```python
from build123d import *

# Parameters (mm, degrees)
F0_W     = 76.2
F0_H     = 50.8
F1_DEPTH = 12.7
F3_DEPTH = 50.801
F5_DEPTH = 76.201
F6_R     = 1.27
F7_DEPTH = 12.701


# Not quite as in the source:
# - a feature names something its author has since deleted; it is built from what else it names


with BuildPart() as f1:
    # F0 (on Top) → F1 (new body)
    with BuildSketch(Plane.XY):
        Rectangle(F0_W, F0_H)
    extrude(amount=F1_DEPTH)

    # F2 (on face) → F3 (cut, through all)
    with BuildSketch(Plane.XZ.offset(25.4)):
        with BuildLine():
            Line((6.4135, 12.7), (-6.4135, 12.7))
            Line((-6.4135, 12.7), (-6.4135, 11.2776))
            ThreePointArc((-6.4135, 11.2776), (-5.7912, 10.6553), (-6.4135, 10.033))
            Line((-6.4135, 10.033), (-6.4135, 8.7376))
            ThreePointArc((-6.4135, 8.7376), (-5.7912, 8.1153), (-6.4135, 7.493))
            Line((-6.4135, 7.493), (-6.4135, 6.223))
            Line((-6.4135, 6.223), (6.4135, 6.223))
            Line((6.4135, 6.223), (6.4135, 7.493))
            ThreePointArc((6.4135, 7.493), (5.7912, 8.1153), (6.4135, 8.7376))
            Line((6.4135, 8.7376), (6.4135, 10.033))
            ThreePointArc((6.4135, 10.033), (5.7912, 10.6553), (6.4135, 11.2776))
            Line((6.4135, 11.2776), (6.4135, 12.7))
        make_face()
    extrude(amount=-F3_DEPTH, mode=Mode.SUBTRACT)

    # F4 (on face) → F5 (cut, through all)
    with BuildSketch(Plane.YZ.offset(38.1)):
        with BuildLine():
            Line((6.4135, 12.7), (-6.4135, 12.7))
            Line((-6.4135, 12.7), (-6.4135, 11.2776))
            ThreePointArc((-6.4135, 11.2776), (-5.7912, 10.6553), (-6.4135, 10.033))
            Line((-6.4135, 10.033), (-6.4135, 8.7376))
            ThreePointArc((-6.4135, 8.7376), (-5.7912, 8.1153), (-6.4135, 7.493))
            Line((-6.4135, 7.493), (-6.4135, 6.223))
            Line((-6.4135, 6.223), (6.4135, 6.223))
            Line((6.4135, 6.223), (6.4135, 7.493))
            ThreePointArc((6.4135, 7.493), (5.7912, 8.1153), (6.4135, 8.7376))
            Line((6.4135, 8.7376), (6.4135, 10.033))
            ThreePointArc((6.4135, 10.033), (5.7912, 10.6553), (6.4135, 11.2776))
            Line((6.4135, 11.2776), (6.4135, 12.7))
        make_face()
    extrude(amount=-F5_DEPTH, mode=Mode.SUBTRACT)

    # F6 (on Top) → F7 (cut, through all)
    with BuildSketch(Plane.XY):
        Circle(F6_R)
    extrude(amount=F7_DEPTH, mode=Mode.SUBTRACT)


solid = f1.part
```
Design review of the part built by this model. Coordinates are the model's own, in mm. A direction names the side the tool comes from. Round coordinates to 2 decimals unless told otherwise and drop trailing zeros. Write each loop counter-clockwise with the first axis right and the second up, starting at its lowest first coordinate (ties: lowest second). Pieces come first, ordered by that corner, then holes.
Item 1: We need section D-D on y = -19. Write out the cut boundary in (x, z), and give its area (3 significant figures).
Item 2: We need section B-B on y = 0. Write out the cut boundary in (x, z), and give its area (3 significant figures).
Item 3: For faces 5 (the flat face through (-38.1, 0, 5)), 6 (the flat face through (-6.414, 16, 12)), 7 (the flat face through (1, 5, 6.223)), 8 (the flat face through (-22, 6.414, 12)), 9 (the flat face through (-1, 6, 0)), list the 3-axis set-ups (+Z, -Z, +X, -X, +Y, -Y) from which the entire face can be reached by the end or side of a thin tool; tool diameter is ignored.
Item 4: We need section A-A on x = 0. Write out the cut boundary in (y, z), and give its area (3 significant figures).
Item 5: For probe 1 along Y at (x, z) = (34.5, 6.5); probe 2 along X at (y, z) = (18.5, 10.75); probe 3 along Y at (x, z) = (-31, 8.25), list the stretches that pass through material, from the lowest coordinate up.
Item 6: The part is to be moulded in two halves that separate along Y. For faces 1 (the flat face through (-22, -6.414, 12)), 2 (the flat face through (6.414, -16, 12)), 3 (the flat face through (22, -6.414, 12)), 4 (the flat face through (-1, -25.4, 5)), say which applies: +Y half, -Y half, draft (parallel to the pull), parting line (faces both ways), or undercut.
Item 7: Clearance check with a flat-ended pin moving along its axis: pin 1 Ø5 at (x, z) = (3.5, 10) entering from +Y. State where the tip first meets the part, or that it passes through.
Item 8: We need section C-C on x = 26. Write out the cut boundary in (y, z), and give its area (3 significant figures).
Returned:
1. outline: (-38.1, 0) - (38.1, 0) - (38.1, 12.7) - (6.41, 12.7) - (6.41, 11.28) arc R0.62 ccw to (6.41, 10.03) - (6.41, 8.74) arc R0.62 ccw to (6.41, 7.49) - (6.41, 6.22) - (-6.41, 6.22) - (-6.41, 7.49) arc R0.62 ccw to (-6.41, 8.74) - (-6.41, 10.03) arc R0.62 ccw to (-6.41, 11.28) - (-6.41, 12.7) - (-38.1, 12.7) - close
1. area: 887 mm2
2. outline: (-38.1, 0) - (-1.27, 0) - (-1.27, 6.22) - (-38.1, 6.22) - close; (1.27, 0) - (38.1, 0) - (38.1, 6.22) - (1.27, 6.22) - close
2. area: 458 mm2
3. face 5: +Z, -Z, -X, +Y, -Y
3. face 6: +Z, +Y, -Y
3. face 7: none
3. face 8: +Z, +X, -X
3. face 9: -Z, +X, -X, +Y, -Y
4. outline: (-25.4, 0) - (-1.27, 0) - (-1.27, 6.22) - (-25.4, 6.22) - close; (1.27, 0) - (25.4, 0) - (25.4, 6.22) - (1.27, 6.22) - close
4. area: 300 mm2
5. probe 1: y = -25.4 to -6.41, 6.41 to 25.4
5. probe 2: x = -38.1 to -5.8, 5.8 to 38.1
5. probe 3: y = -25.4 to -5.81, 5.81 to 25.4
6. face 1: undercut
6. face 2: draft
6. face 3: undercut
6. face 4: -Y half
7. pin 1: stops at y = 25.4
8. outline: (-25.4, 0) - (25.4, 0) - (25.4, 12.7) - (6.41, 12.7) - (6.41, 11.28) arc R0.62 ccw to (6.41, 10.03) - (6.41, 8.74) arc R0.62 ccw to (6.41, 7.49) - (6.41, 6.22) - (-6.41, 6.22) - (-6.41, 7.49) arc R0.62 ccw to (-6.41, 8.74) - (-6.41, 10.03) arc R0.62 ccw to (-6.41, 11.28) - (-6.41, 12.7) - (-25.4, 12.7) - close
8. area: 565 mm2
